from build123d import *

# Parameters (mm, degrees)
CROQUIS1_R              = 12
SALIENTE_EXTRUIR1_DEPTH = 5
CROQUIS2_R              = 1.7
CORTAR_EXTRUIR1_DEPTH   = 5
CROQUIS3_R              = 2.95
CORTAR_EXTRUIR2_DEPTH   = 3


with BuildPart() as part:
    # Croquis1 → Saliente-Extruir1 (new body)
    with BuildSketch(Plane(origin=(0, 0, 0), x_dir=(1, 0, 0), z_dir=(0, 1, 0))):
        with BuildLine():
            ThreePointArc((-12.848290026, -59.631547384), (0, -61), (12.848290026, -59.631547384))
            ThreePointArc((12.848290026, -59.631547384), (14.396355702, -58.025376654), (13.494442308, -55.985071779))
            ThreePointArc((13.494442308, -55.985071779), (14.829055081, -29.865027209), (36.444464672, -44.589564139))
            ThreePointArc((36.444464672, -44.589564139), (37.524744291, -46.541303798), (39.740011147, -46.278845211))
            ThreePointArc((39.740011147, -46.278845211), (0, 61), (-39.740011147, -46.278845211))
            ThreePointArc((-39.740011147, -46.278845211), (-37.524744291, -46.541303798), (-36.444464672, -44.589564139))
            ThreePointArc((-36.444464672, -44.589564139), (-14.829055081, -29.865027209), (-13.494442308, -55.985071779))
            ThreePointArc((-13.494442308, -55.985071779), (-14.396355702, -58.025376654), (-12.848290026, -59.631547384))
        make_face()
        Circle(CROQUIS1_R, mode=Mode.SUBTRACT)
    extrude(amount=SALIENTE_EXTRUIR1_DEPTH)

    # Croquis2 → Cortar-Extruir1 (cut)
    with BuildSketch(Plane(origin=(0, 5, 0), x_dir=(1, 0, 0), z_dir=(0, 1, 0))):
        with Locations((-15.5, 15.5)):
            Circle(CROQUIS2_R)
        with Locations((-15.5, -15.5)):
            Circle(CROQUIS2_R)
        with Locations((15.5, -15.5)):
            Circle(CROQUIS2_R)
        with Locations((15.5, 15.5)):
            Circle(CROQUIS2_R)
        with BuildLine():
            Line((-34.8, -26.3), (-34.8, -29.3))
            ThreePointArc((-34.8, -29.3), (-36.5, -31), (-38.2, -29.3))
            Line((-38.2, -29.3), (-38.2, -26.3))
            ThreePointArc((-38.2, -26.3), (-36.5, -24.6), (-34.8, -26.3))
        make_face()
        with BuildLine():
            Line((-4.8, -26.3), (-4.8, -29.3))
            ThreePointArc((-4.8, -29.3), (-6.5, -31), (-8.2, -29.3))
            Line((-8.2, -29.3), (-8.2, -26.3))
            ThreePointArc((-8.2, -26.3), (-6.5, -24.6), (-4.8, -26.3))
        make_face()
        with BuildLine():
            Line((4.8, -26.3), (4.8, -29.3))
            ThreePointArc((4.8, -29.3), (6.5, -31), (8.2, -29.3))
            Line((8.2, -29.3), (8.2, -26.3))
            ThreePointArc((8.2, -26.3), (6.5, -24.6), (4.8, -26.3))
        make_face()
        with BuildLine():
            Line((34.8, -26.3), (34.8, -29.3))
            ThreePointArc((34.8, -29.3), (36.5, -31), (38.2, -29.3))
            Line((38.2, -29.3), (38.2, -26.3))
            ThreePointArc((38.2, -26.3), (36.5, -24.6), (34.8, -26.3))
        make_face()
    extrude(amount=-CORTAR_EXTRUIR1_DEPTH, mode=Mode.SUBTRACT)

    # Croquis3 → Cortar-Extruir2 (cut)
    with BuildSketch(Plane(origin=(0, 5, 0), x_dir=(1, 0, 0), z_dir=(0, 1, 0))):
        with Locations((-15.5, 15.5)):
            Circle(CROQUIS3_R)
        with Locations((15.5, 15.5)):
            Circle(CROQUIS3_R)
        with Locations((15.5, -15.5)):
            Circle(CROQUIS3_R)
        with Locations((-15.5, -15.5)):
            Circle(CROQUIS3_R)
        with BuildLine():
            Line((-33.55, -26.3), (-33.55, -29.3))
            ThreePointArc((-33.55, -29.3), (-36.5, -32.25), (-39.45, -29.3))
            Line((-39.45, -29.3), (-39.45, -26.3))
            ThreePointArc((-39.45, -26.3), (-36.5, -23.35), (-33.55, -26.3))
        make_face()
        with BuildLine():
            Line((-3.55, -26.3), (-3.55, -29.3))
            ThreePointArc((-3.55, -29.3), (-6.5, -32.25), (-9.45, -29.3))
            Line((-9.45, -29.3), (-9.45, -26.3))
            ThreePointArc((-9.45, -26.3), (-6.5, -23.35), (-3.55, -26.3))
        make_face()
        with BuildLine():
            Line((9.45, -26.3), (9.45, -29.3))
            ThreePointArc((9.45, -29.3), (6.5, -32.25), (3.55, -29.3))
            Line((3.55, -29.3), (3.55, -26.3))
            ThreePointArc((3.55, -26.3), (6.5, -23.35), (9.45, -26.3))
        make_face()
        with BuildLine():
            Line((39.45, -26.3), (39.45, -29.3))
            ThreePointArc((39.45, -29.3), (36.5, -32.25), (33.55, -29.3))
            Line((33.55, -29.3), (33.55, -26.3))
            ThreePointArc((33.55, -26.3), (36.5, -23.35), (39.45, -26.3))
        make_face()
    extrude(amount=-CORTAR_EXTRUIR2_DEPTH, mode=Mode.SUBTRACT)


solid = part.part
Geometry: final body of the model. Coordinates: model frame, mm. A direction names the side the tool comes from. Round coordinates to 2 decimals unless told otherwise and drop trailing zeros. Write each loop counter-clockwise with the first axis right and the second up, starting at its lowest first coordinate (ties: lowest second). Pieces come first, ordered by that corner, then holes. Notation, with made-up numbers: M 74,67 L 133,67 A22 cw 133,102 Z; hole C 33,32 d9. An arc over 180 degrees is marked long. Write item = value, one per line.
Item 1: Access query for faces 1 (the face through (39.45, 4, 28)), 2 (the face through (-13.93, 1.01, 16.15)). Directions: +Z, -Z, +X, -X, +Y, -Y. A direction counts if a zero-diameter tool reaches every point of the face in a straight line with its end or side. Return the directions, or none.
Findings:
face_1 = +Y
face_2 = +Y, -Y
Item 2: Section query B-B on y = 3.7. State how many separate pieces and enclosed holes the cut face has, then the cut area to 3 significant figures.
Findings:
separate_pieces = 1
enclosed_holes = 9
area = 9,570 mm^2
Item 3: Section query D-D on x = -21.5. Return loops of the section in (y, z).
Findings:
outline = M 0,-57.09 L 5,-57.09 L 5,28.3 L 0,28.3 Z
Item 4: Pull-direction query (X, two-part tool) for faces 3 (the face through (14.39, 2.46, 58.06)), 4 (the face through (12.553, 3.521, -15.63)), 5 (the face through (-14, 2, -14)); classes: pulls with the +X half, pulls with the -X half, needs draft (parallel to the pull), parting line crosses it, or undercut.
Findings:
face_3 = pulls with the +X half
face_4 = undercut
face_5 = undercut
Item 5: Section query A-A on z = 0. Return loops of the section in (x, y).
Findings:
outline = M -61,0 L -12,0 L -12,5 L -61,5 Z; M 12,0 L 61,0 L 61,5 L 12,5 Z
Item 6: Section query C-C on z = 15.5. Return loops of the section in (x, y).
Findings:
outline = M -59,0 L -17.2,0 L -17.2,2 L -18.45,2 L -18.45,5 L -59,5 Z; M -13.8,0 L 13.8,0 L 13.8,2 L 12.55,2 L 12.55,5 L -12.55,5 L -12.55,2 L -13.8,2 Z; M 17.2,0 L 59,0 L 59,5 L 18.45,5 L 18.45,2 L 17.2,2 Z
Item 7: Pin query (flat end, axial travel): P1, Ø5.5, axis at x = 15.5, z = -15.5, coming from the +Y side; P2, Ø4.5, axis at x = -15.5, z = -15.5, coming from the -Y side; P3, Ø1.5, axis at y = 3.5, z = 27.5, coming from the +X side; P4, Ø2, axis at x = 15.5, z = -15.5, coming from the +Y side. Return the tip coordinate at first contact, or that it passes through.
Findings:
P1 = 2
P2 = 0
P3 = 54.82
P4 = through
Item 8: Material intervals for line 1 along X through (y, z) = (2.4, -17); line 2 along Z through (x, y) = (-15.5, 2.95); line 3 along X through (y, z) = (4.05, 15.5), sorted ascending. Write a range as [from, to].
Findings:
line_1 = [-58.58, -18.04], [-12.96, 12.96], [18.04, 58.58]
line_2 = [-59, -18.45], [-12.55, 12.55], [18.45, 29.55]
line_3 = [-59, -18.45], [-12.55, 12.55], [18.45, 59]
